```python
from build123d import *

# Parameters (mm, degrees)
SKETCH_1_R          = 1.025
SKETCH_1_R_2        = 1.5
SKETCH_1_R_3        = 1.125
EXTRUDE_1_DEPTH     = 6
SKETCH_3_R          = 2.5
CUT_EXTRUDE_1_DEPTH = 3
FILLET_1_R          = 4


with BuildPart() as part:
    # 草图1 → 凸台-拉伸1 (new body)
    with BuildSketch(Plane(origin=(0, 0, 0), x_dir=(1, 0, 0), z_dir=(0, 1, 0))):
        with BuildLine():
            Line((0, -3.5), (15.612494996, -3.5))
            ThreePointArc((15.612494996, -3.5), (11.313708499, 11.313708499), (-3.5, 15.612494996))
            Line((-3.5, 15.612494996), (-3.5, 0))
            ThreePointArc((-3.5, 0), (-2.474873734, -2.474873734), (0, -3.5))
        make_face()
        with Locations((8.5, 0)):
            Circle(SKETCH_1_R, mode=Mode.SUBTRACT)
        with Locations((13.5, 0)):
            Circle(SKETCH_1_R, mode=Mode.SUBTRACT)
        Circle(SKETCH_1_R_2, mode=Mode.SUBTRACT)
        with Locations((0, 12)):
            Circle(SKETCH_1_R_3, mode=Mode.SUBTRACT)
        with Locations((0, 8)):
            Circle(SKETCH_1_R_3, mode=Mode.SUBTRACT)
        with Locations((0, 5)):
            Circle(SKETCH_1_R_3, mode=Mode.SUBTRACT)
    extrude(amount=EXTRUDE_1_DEPTH)

    # 草图3 → 切除-拉伸1 (cut)
    with BuildSketch(Plane.XZ):
        Circle(SKETCH_3_R)
    extrude(amount=-CUT_EXTRUDE_1_DEPTH, mode=Mode.SUBTRACT)

    # 圆角1
    fillet_1_edges = [part.edges().sort_by_distance(p)[0] for p in [
        (15.612494996, 3, 3.5),
        (-3.5, 3, -15.612494996),
    ]]
    fillet(fillet_1_edges, radius=FILLET_1_R)


solid = part.part
```
The model under review builds one solid part; all positions refer to its coordinate system, in mm. A direction names the side the tool comes from. Give positions to 0.01 mm unless a question says otherwise; leave off trailing zeros. Write each loop counter-clockwise with the first axis right and the second up, starting at its lowest first coordinate (ties: lowest second). Pieces come first, ordered by that corner, then holes.
(1) The part is to be moulded in two halves that separate along X. For faces 3 (the cylindrical face through (-1.5, 4.48, -0.07)), 4 (the flat face through (6, 3, 3.5)), 5 (the flat face through (-3.5, 3, -6)), say which applies: released by +X, released by -X, zero draft, split by the parting line, or undercut.
(2) Tool access review of faces 1 (the flat face through (0, 3, -2)), 2 (the cylindrical face through (11.431, 2.958, -11.195)): name each direction out of +Z, -Z, +X, -X, +Y, -Y from which nothing blocks a thin tool from reaching the whole face with its end or side.
(3) Consider section C-C, the plane x = 13.5. Give the boundary of the cut face in (y, z) (3 decimals), and give its area (4 significant figures).
(4) To check wall thickness, follow L1, parallel to X at y = 1.9, z = 0.25; L2, parallel to Z at x = 1, y = 5.05; L3, parallel to Z at x = 0, y = 4.75 (3 decimals). State the ranges of each line that lie inside material, in increasing order.
(5) Consider section D-D, the plane y = 1.3. Give the boundary of the cut face in (x, z) (3 decimals), and give its area (3 significant figures).
(6) For P1, Ø1.8, axis at x = 0, z = 0, coming from the -Y side; P2, Ø2, axis at x = 13.5, y = 4, coming from the -Z side; P3, Ø1, axis at y = 1.5, z = -2.5, coming from the +X side, all flat-tipped, find the tip position at first contact; note any pin that passes through.
(7) Consider section A-A, the plane y = 4.6. Give the boundary of the cut face in (x, z) (3 decimals).
(8) Consider section B-B, the plane z = -11.75. Give the boundary of the cut face in (x, y).
Returned:
1. face 3: undercut
1. face 4: zero draft
1. face 5: released by -X
2. face 1: -Y
2. face 2: -Z, +X, +Y, -Y
3. outline: (0, -8.588) - (6, -8.588) - (6, -1.025) - (0, -1.025) - close; (0, 1.025) - (6, 1.025) - (6, 3.204) - (0, 3.204) - close
3. area: 58.45 mm2
4. L1: x = -3.49 to -2.49, 2.49 to 7.51, 9.49 to 12.51, 14.49 to 15.92
4. L2: z = -15.97 to -12.52, -11.48 to -8.52, -7.48 to -5.52, -4.48 to -1.12, 1.12 to 3.5
4. L3: z = -15.958 to -13.125, -10.875 to -9.125, -6.875 to -6.125, -3.875 to -1.5, 1.5 to 3.5
5. outline: (-3.5, -11.99) arc R4 ccw to (0.667, -15.986) arc R16 ccw to (15.986, -0.667) arc R4 ccw to (11.99, 3.5) - (0, 3.5) arc R3.5 ccw to (-3.5, 0) - close; hole circle Ø5 at (0, 0); hole circle Ø2.25 at (0, -12); hole circle Ø2.25 at (0, -8); hole circle Ø2.25 at (0, -5); hole circle Ø2.05 at (8.5, 0); hole circle Ø2.05 at (13.5, 0)
5. area: 278 mm2
6. P1: passes through
6. P2: stops at z = -9.99
6. P3: stops at x = 15.87
7. outline: (-3.5, -11.99) arc R4 ccw to (0.667, -15.986) arc R16 ccw to (15.986, -0.667) arc R4 ccw to (11.99, 3.5) - (0, 3.5) arc R3.5 ccw to (-3.5, 0) - close; hole circle Ø3 at (0, 0); hole circle Ø2.25 at (0, -12); hole circle Ø2.25 at (0, -8); hole circle Ø2.25 at (0, -5); hole circle Ø2.05 at (8.5, 0); hole circle Ø2.05 at (13.5, 0)
8. outline: (-3.5, 0) - (-1.1, 0) - (-1.1, 6) - (-3.5, 6) - close; (1.1, 0) - (10.86, 0) - (10.86, 6) - (1.1, 6) - close
